Build history of the part. All positions in model axes, mm. A direction names the side the tool comes from. Round coordinates to 2 decimals unless told otherwise and drop trailing zeros. Write each loop counter-clockwise with the first axis right and the second up, starting at its lowest first coordinate (ties: lowest second). Pieces come first, ordered by that corner, then holes.
Item 1: Band-saw the part on B-B, the plane y = -11. Write the cut outline in (x, z), then the cut area to 3 significant figures.
Item 2: 3-axis set-ups, long thin cutter, end or side, ignore diameter. For faces 4 (the flat face through (-24.713, -4, 4)), 5 (the flat face through (23, -20.266, 4)), 6 (the flat face through (23, 13.734, 4)), 7 (the flat face through (-16.813, 20, 4)), 8 (the flat face through (0, 16, 1.648)): which of +Z, -Z, +X, -X, +Y, -Y reach the whole face in a straight line?
Item 3: Mould opens along Z. For faces 1 (the flat face through (-11, -14, 8)), 2 (the cylindrical face through (6.725, 15.812, 5.293)), 3 (the flat face through (-23, -20.266, 4)) say: +Z half, -Z half, draft (parallel to the pull), parting line (faces both ways), or undercut.
Item 4: Wall check: probe 1 along Z at (x, y) = (-1, 12.5); probe 2 along Y at (x, z) = (-2, 2); probe 3 along X at (y, z) = (15, 5). Give the ranges that are in metal, low to high.
Item 5: Band-saw the part on A-A, the plane x = 14. Write the cut outline in (y, z), then the cut area to 3 significant figures.
Item 6: Drop flat-ended pins along their axis: pin 1 Ø9.5 at (x, y) = (-3.5, 15.5) entering from +Z; pin 2 Ø3 at (y, z) = (20, 2) entering from -X; pin 3 Ø1.1 at (x, z) = (-23, 4) entering from +Y; pin 4 Ø1.9 at (x, z) = (23.5, 5) entering from -Y. Give the stop position or say it passes through.
Item 7: Band-saw the part on C-C, the plane z = 1. Write the cut outline in (x, y).
Item 8: Band-saw the part on D-D, the plane z = 5.5. Write the cut outline in (x, y).
Autodesk Inventor part; units mm, degrees
ref_plane "YZ Plane" through (0, 0, 0) normal (1, 0, 0) x (0, 1, 0)
ref_plane "XZ Plane" through (0, 0, 0) normal (0, 1, 0) x (-1, 0, 0)
ref_plane "XY Plane" through (0, 0, 0) normal (0, 0, 1) x (1, 0, 0)
sketch "Sketch1" plane through (0, 0, 0) normal (0, 0, 1) x (1, 0, 0)
  line L0 (21.5871, 13.6345) -> (17.0871, 18.1345)
  line L1 (17.0871, 18.1345) -> (-16.7129, 18.1345)
  line L2 (-16.7129, 18.1345) -> (-21.2129, 13.6345)
  line L3 (-21.0966, 13.6345) -> (-21.0966, -20.1655)
  line L4 (21.4709, -20.1655) -> (21.4709, 13.6345)
  line L5 (21.4709, -20.1655) -> (17.0871, -24.4078)
  line L6 (-16.7129, -24.4078) -> (17.0871, -24.4078)
  line L7 (-16.7129, -24.4078) -> (-21.0966, -20.1655)
  line L8 (-24.7129, -28.1655) -> (-24.7129, 13.6345) construction
  line L9 (25.0871, -28.1655) -> (-24.7129, -28.1655) construction
  line L10 (25.0871, -28.1655) -> (25.0871, 13.6345) construction
  line L11 (17.0871, 21.6345) -> (-16.7129, 21.6345) construction
  line L12 (-21.0552, -20.0655) -> (-16.6129, -24.5078)
  line L13 (-16.6129, -24.5078) -> (-16.6129, -28.1655)
  line L14 (-16.6129, -28.1655) -> (17.0871, -28.1655)
  line L15 (25.0871, -20.0655) -> (21.4295, -20.0655)
  line L16 (25.0871, 13.5345) -> (25.0871, -20.0655)
  line L17 (21.4295, 13.5345) -> (25.0871, 13.5345)
  line L18 (21.4295, 13.5345) -> (16.9871, 17.9768)
  line L19 (16.9871, 17.9768) -> (16.9871, 21.6345)
  line L20 (16.9871, 21.6345) -> (-16.6129, 21.6345)
  line L21 (-16.6129, 21.6345) -> (-16.6129, 17.9768)
  line L22 (-16.6129, 17.9768) -> (-21.0552, 13.5345)
  line L23 (-24.7129, 13.5345) -> (-21.0552, 13.5345)
  line L24 (-24.7129, -20.0655) -> (-24.7129, 13.5345)
  line L25 (-21.0552, -20.0655) -> (-24.7129, -20.0655)
  line L26 (-12.3129, -23.2655) -> (12.6871, -23.2655)
  line L27 (12.6871, -23.2655) -> (12.6871, 16.7345)
  line L28 (-12.3129, 16.7345) -> (12.6871, 16.7345)
  line L29 (-12.3129, -23.2655) -> (-12.3129, 16.7345)
  line L30 (14.6871, -25.2655) -> (-14.3129, -25.2655) construction
  line L31 (-14.3129, -25.2655) -> (-14.3129, 18.7345) construction
  line L32 (-14.3129, 18.7345) -> (14.6871, 18.7345) construction
  line L33 (14.6871, 18.7345) -> (14.6871, -25.2655) construction
  line L34 (-17.3129, 21.7345) -> (17.6871, 21.7345) construction
  line L35 (17.6871, 21.7345) -> (17.6871, -28.2655) construction
  line L36 (17.6871, -28.2655) -> (-17.3129, -28.2655) construction
  line L37 (-17.3129, -28.2655) -> (-17.3129, 21.7345) construction
  line L38 (-14.3129, -23.2655) -> (-14.3129, -25.2655)
  line L39 (-14.3129, -25.2655) -> (14.6871, -25.2655)
  line L40 (14.6871, -25.2655) -> (14.6871, -20.0655)
  line L41 (14.6871, -20.0655) -> (17.6871, -20.0655)
  line L42 (17.6871, -20.0655) -> (17.6871, 13.5345)
  line L43 (17.6871, 13.5345) -> (14.6871, 13.5345)
  line L44 (14.6871, 13.5345) -> (14.6871, 18.7345)
  line L45 (14.6871, 18.7345) -> (-14.3129, 18.7345)
  line L46 (-14.3129, 18.7345) -> (-14.3129, 13.5345)
  line L47 (-14.3129, 13.5345) -> (-17.3129, 13.5345)
  line L48 (-17.3129, 13.5345) -> (-17.3129, -20.0655)
  line L49 (-17.3129, -20.0655) -> (-14.3129, -20.0655)
  line L50 (-14.3129, -20.0655) -> (-14.3129, -23.2655)
  line L51 (-16.6129, -28.1655) -> (17.0871, -28.1655)
  line L52 (16.9871, -28.1655) -> (16.9871, -24.3509)
  line L53 (16.9871, -24.3509) -> (21.2726, -20.0655)
  line L54 (21.2726, -20.0655) -> (21.4295, -20.0655)
  point P0 (14.2, -44.8454)
  point P1 (16.9871, 19.8057)
  dimension "d74" = 2
  dimension "d75" = 5
  dimension "d76" = 135
extrude "Extrusion1" add sketch "Sketch1" along normal blind 8 contours L19 L18 L17 L4 L15 L54 L53 L52 L6 L40 L41 L42 L43 L44 L1 | L1 L44 L45 L46 L21 L20 L19 | L44 L43 L42 L41 L40 L6 L38 L50 L49 L48 L47 L46 L1 | L1 L46 L45 L44 | L46 L47 L48 L49 L50 L38 L6 L12 L25 L3 L23 L22 L21 L1 | L17 L16 L15 L4 | L3 L25 L24 L23 | L40 L39 L38 L6 | L6 L52 L14 L13 L12 L38 L39 L40 | L29 L28 L27 L26
sketch "Skizze7" plane through (0, 0, 8) normal (0, 0, 1) x (1, 0, 0)
  line L0 (-21.0552, -20.0655) -> (-16.6129, -24.5078)
  line L1 (-16.6129, -24.5078) -> (-16.6129, -28.1655)
  line L2 (-16.6129, -28.1655) -> (16.9871, -28.1655) construction
  line L3 (16.9871, -28.1655) -> (16.9871, -24.3509)
  line L4 (16.9871, -24.3509) -> (21.2726, -20.0655)
  line L5 (21.2726, -20.0655) -> (25.0871, -20.0655)
  line L6 (25.0871, -20.0655) -> (25.0871, 13.5345) construction
  line L7 (25.0871, 13.5345) -> (21.4295, 13.5345)
  line L8 (21.4295, 13.5345) -> (16.9871, 17.9768)
  line L9 (16.9871, 17.9768) -> (16.9871, 21.6345)
  line L10 (16.9871, 21.6345) -> (-16.6129, 21.6345) construction
  line L11 (-16.6129, 21.6345) -> (-16.6129, 17.9768)
  line L12 (-16.6129, 17.9768) -> (-21.0552, 13.5345)
  line L13 (-21.0552, 13.5345) -> (-24.7129, 13.5345)
  line L14 (-24.7129, 13.5345) -> (-24.7129, -20.0655) construction
  line L15 (-24.7129, -20.0655) -> (-21.0552, -20.0655)
  line L16 (-16.8129, 21.8345) -> (17.1871, 21.8345) construction
  line L17 (17.1871, 21.8345) -> (17.1871, 18.0597)
  line L18 (17.1871, 18.0597) -> (21.5123, 13.7345)
  line L19 (21.5123, 13.7345) -> (25.2871, 13.7345)
  line L20 (25.2871, 13.7345) -> (25.2871, -20.2655) construction
  line L21 (25.2871, -20.2655) -> (21.3554, -20.2655)
  line L22 (21.3554, -20.2655) -> (17.1871, -24.4338)
  line L23 (17.1871, -24.4338) -> (17.1871, -28.3655)
  line L24 (17.1871, -28.3655) -> (-16.8129, -28.3655) construction
  line L25 (-16.8129, -28.3655) -> (-16.8129, -24.5907)
  line L26 (-16.8129, -24.5907) -> (-21.1381, -20.2655)
  line L27 (-21.1381, -20.2655) -> (-24.9129, -20.2655)
  line L28 (-24.9129, -20.2655) -> (-24.9129, 13.7345) construction
  line L29 (-24.9129, 13.7345) -> (-21.1381, 13.7345)
  line L30 (-21.1381, 13.7345) -> (-16.8129, 18.0597)
  line L31 (-16.8129, 18.0597) -> (-16.8129, 21.8345)
  line L32 (-21.0552, 13.5345) -> (-24.7129, 13.5345)
  line L33 (-24.7129, 13.5345) -> (-24.7129, 13.7345)
  line L34 (-16.6129, 21.6345) -> (-16.6129, 17.9768)
  line L35 (-16.6129, 21.6345) -> (-16.8129, 21.6345)
  line L36 (25.0871, -20.0655) -> (25.0871, 13.5345)
  line L37 (25.0871, 13.5345) -> (25.0871, 13.7345)
  line L38 (16.9871, 21.6345) -> (17.1871, 21.6345)
  line L39 (16.9871, -28.1655) -> (17.1871, -28.1655)
  line L40 (25.0871, -20.0655) -> (25.0871, -20.2655)
  line L41 (-16.6129, -28.1655) -> (-16.8129, -28.1655)
  line L42 (-24.7129, -20.0655) -> (-24.7129, -20.2655)
  dimension "d94" = 0.2
extrude "IM_offset" add sketch "Skizze7" against normal up to surface (8 mm away)
sketch "Sketch8" plane through (-16.8129, 21.6345, 0) normal (0, 1, 0) x (1, 0, 0)
  line L0 (0, 0) -> (34, 0)
  line L1 (34, -8) -> (0, -8)
  line L2 (9.1629, -1.6478) -> (24.4629, -1.6478)
  arc A0 (9.1629, -1.6478) -> (24.4629, -1.6478) centre (16.8129, -1.6478) ccw
  line L3 (0, -8) -> (0, 0)
  line L4 (34, -8) -> (34, 0)
  point P0 (16.8129, 0)
  dimension "d86" = 15.3
  dimension "d88" = 0
extrude "Extrusion7" cut sketch "Sketch8" against normal blind 45 contours A0 L2 L1 | L1 A0
sketch "Sketch9" plane through (0, 0, 8) normal (0, 0, 1) x (1, 0, 0)
  line L0 (-4.2628, 21.6345) -> (-16.8129, 21.6345)
  line L1 (-24.7129, 13.7345) -> (-24.7129, -20.2655)
  line L2 (17.1871, -28.1655) -> (-16.8129, -28.1655)
  line L3 (25.0871, -20.0655) -> (25.0871, 13.7345)
  circle A0 centre (0.1871, -3.187) radius 27.0445
  circle A1 centre (0.1871, -3.187) radius 15
  line L4 (4.2628, 21.6345) -> (4.2628, -23.3655)
  line L5 (4.2628, -23.3655) -> (-4.2628, -23.3655)
  line L6 (-4.2628, -23.3655) -> (-4.2628, 21.6345)
  line L7 (17.1871, 21.6345) -> (4.2628, 21.6345)
  line L8 (-16.8129, 21.6345) -> (-16.8129, 18.0597)
  line L9 (-16.8129, 18.0597) -> (-21.1381, 13.7345)
  line L10 (-21.1381, 13.7345) -> (-24.7129, 13.7345)
  line L11 (17.1871, -28.1655) -> (17.1871, -24.4338)
  line L12 (17.1871, -24.4338) -> (21.3554, -20.2655)
  line L13 (21.3554, -20.2655) -> (25.0871, -20.2655)
  line L14 (25.0871, -20.2655) -> (25.0871, -20.0655)
  line L15 (25.0871, 13.7345) -> (21.5123, 13.7345)
  line L16 (21.5123, 13.7345) -> (17.1871, 18.0597)
  line L17 (17.1871, 18.0597) -> (17.1871, 21.6345)
  line L18 (-21.1381, -20.2655) -> (-24.7129, -20.2655)
  line L19 (-16.8129, -24.5907) -> (-21.1381, -20.2655)
  line L20 (-16.8129, -28.1655) -> (-16.8129, -24.5907)
  point P0 (0, 0)
  dimension "d91" = 30
extrude "Extrusion8" cut sketch "Sketch9" against normal through all contours L6 A1 | A1 L4 L6 | A1 L4
properties part number "20_Cube_Insert_Lens_Cylindrical_Plexiglas_glassslab_v3"
Results:
1. outline: (-24.71, 0) - (-12.62, 0) - (-12.62, 8) - (-24.71, 8) - close; (12.99, 0) - (25.09, 0) - (25.09, 8) - (12.99, 8) - close
1. area: 194 mm2
2. face 4: +Z, -Z, -X, +Y, -Y
2. face 5: +Z, -Z, +X, -Y
2. face 6: +Z, -Z, +X, +Y
2. face 7: +Z, -Z, -X, +Y
2. face 8: +Y
3. face 1: +Z half
3. face 2: undercut
3. face 3: draft
4. probe 1: z = 0 to 1.65
4. probe 2: y = -28.17 to -23.37
4. probe 3: x = -19.87 to -6.88, 6.88 to 20.25
5. outline: (-28.17, 0) - (-9.04, 0) - (-9.04, 8) - (-28.17, 8) - close; (2.66, 0) - (21.63, 0) - (21.63, 8) - (2.66, 8) - close
5. area: 305 mm2
6. pin 1: stops at z = 8
6. pin 2: stops at x = -16.81
6. pin 3: stops at y = 13.73
6. pin 4: stops at y = -20.27
7. outline: (-24.71, -20.27) - (-21.14, -20.27) - (-16.81, -24.59) - (-16.81, -28.17) - (17.19, -28.17) - (17.19, -24.43) - (21.36, -20.27) - (25.09, -20.27) - (25.09, 13.73) - (21.51, 13.73) - (17.19, 18.06) - (17.19, 21.63) - (-16.81, 21.63) - (-16.81, 18.06) - (-21.14, 13.73) - (-24.71, 13.73) - close; hole circle Ø30 at (0.19, -3.19)
8. outline: (-24.71, -20.27) - (-21.14, -20.27) - (-16.81, -24.59) - (-16.81, -28.17) - (17.19, -28.17) - (17.19, -24.43) - (21.36, -20.27) - (25.09, -20.27) - (25.09, 13.73) - (21.51, 13.73) - (17.19, 18.06) - (17.19, 21.63) - (6.61, 21.63) - (6.61, 10.37) arc R15 cw to (6.61, -16.74) - (6.61, -23.37) - (-6.61, -23.37) - (-6.61, -16.56) arc R15 cw to (-6.61, 10.18) - (-6.61, 21.63) - (-16.81, 21.63) - (-16.81, 18.06) - (-21.14, 13.73) - (-24.71, 13.73) - close
